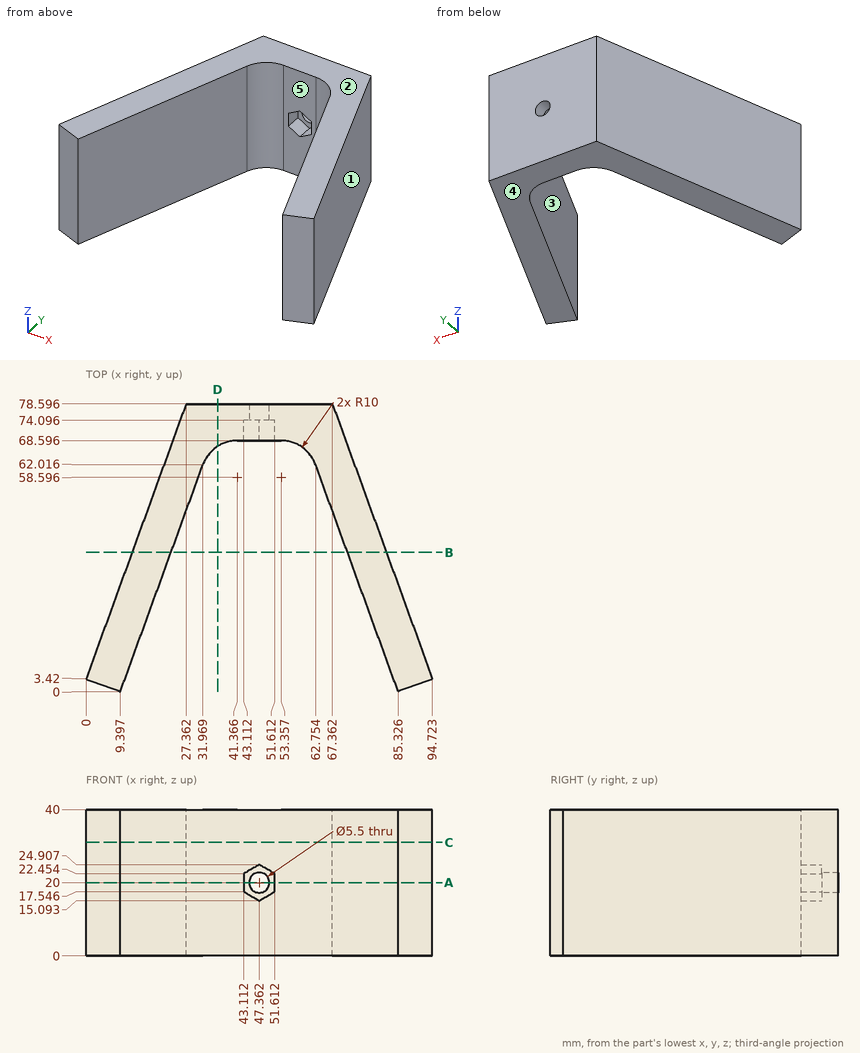
The figure shows three views and two pictorial views of one solid part (mm, origin at its lowest corner). Answer the questions. A direction names the side the tool comes from. Round coordinates to 2 decimals unless told otherwise and drop trailing zeros. Loops run counter-clockwise (first coordinate to the right, second up) from the corner with the lowest first, then second, coordinate; pieces in that order, holes last. Notation, with made-up numbers: (-30.5, 5) - (-24.5, 5) arc R13 ccw to (-24.5, 30) - close; hole circle Ø4 at (13.25, 49). An arc over 180 degrees is marked (long way). Use one line per item in the form item = value. Start each with the question number.
(1) Find section C-C on z = 31. Determine the outline of the cut face in (x, y) (1 decimal), and give its area (3 significant figures).
(2) Which of the six approach directions +Z, -Z, +X, -X, +Y, -Y give full straight-line access (tool end or side, diameter ignored) to the marked faces 4 and 5?
(3) Consider line 1 (X direction, y = 38.5, z = 36.5) (1 decimal); line 2 (X direction, y = 60.5, z = 21) (1 decimal); line 3 (Y direction, x = 40.5, z = 34) (1 decimal). Determine where each line is inside the solid, lowest interval first.
(4) Flat-ended cylindrical pins translate along their axes: P1, Ø5, axis at y = 50, z = 8, coming from the -X side; P2, Ø2.5, axis at y = 71.5, z = 19, coming from the +X side; P3, Ø3, axis at y = 63.5, z = 35, coming from the -X side; P4, Ø1, axis at x = 73, y = 32, coming from the -Z side. Find the tip coordinate at first contact, or state that the pin passes through.
(5) Determine the mould class of the marked faces 1, 2 and 3 for opening direction X: +X half, -X half, draft (parallel to the pull), parting line (faces both ways), or undercut.
(6) Find section B-B on y = 38. Determine the outline of the cut face in (x, z) (1 decimal).
(7) Find section D-D on x = 36. Determine the outline of the cut face in (y, z) (1 decimal).
(8) Find section A-A on z = 20. Determine the outline of the cut face in (x, y) (1 decimal), and give its area (3 significant figures).
Answer list:
q1.outline = (0, 3.4) - (9.4, 0) - (32, 62) arc R10 cw to (41.4, 68.6) - (53.4, 68.6) arc R10 cw to (62.8, 62) - (85.3, 0) - (94.7, 3.4) - (67.4, 78.6) - (27.4, 78.6) - close
q1.area = 1,880 mm^2
q2.face_4 = -Z, +X, -X, +Y, -Y
q2.face_5 = +Z, -Z, -Y
q3.line_1 = 12.8 to 23.4, 71.3 to 82
q3.line_2 = 20.8 to 31.4, 63.3 to 73.9
q3.line_3 = 68.6 to 78.6
q4.P1 = 16.04
q4.P2 = 70.4
q4.P3 = 21.32
q4.P4 = through
q5.face_1 = +X half
q5.face_2 = draft
q5.face_3 = undercut
q6.outline = (12.6, 0) - (23.2, 0) - (23.2, 40) - (12.6, 40) - close; (71.5, 0) - (82.1, 0) - (82.1, 40) - (71.5, 40) - close
q7.outline = (67, 0) - (78.6, 0) - (78.6, 40) - (67, 40) - close
q8.outline = (0, 3.4) - (9.4, 0) - (32, 62) arc R10 cw to (41.4, 68.6) - (43.1, 68.6) - (43.1, 74.1) - (44.6, 74.1) - (44.6, 78.6) - (27.4, 78.6) - close; (50.1, 74.1) - (51.6, 74.1) - (51.6, 68.6) - (53.4, 68.6) arc R10 cw to (62.8, 62) - (85.3, 0) - (94.7, 3.4) - (67.4, 78.6) - (50.1, 78.6) - close
q8.area = 1,810 mm^2
